```python
from build123d import *

# Parameters (mm, degrees)
EXTRUDE_1_DEPTH     = 10
SKETCH_4_R          = 5.17
CUT_EXTRUDE_1_DEPTH = 10
CHAMFER_1_SIZE      = 0.83


with BuildPart() as part:
    # Эскиз1 → Бобышка-Вытянуть1 (new body)
    with BuildSketch(Plane(origin=(0, 0, 0), x_dir=(1, 0, 0), z_dir=(0, 1, 0))):
        Polygon((-5.484827557, 9.5), (-10.969655115, 0), (-5.484827557, -9.5), (5.484827557, -9.5), (10.969655115, 0), (5.484827557, 9.5), align=None)
    extrude(amount=EXTRUDE_1_DEPTH)

    # Эскиз2 → Вырез-Повернуть1 (revolve, cut)
    with BuildSketch(Plane(origin=(0, 0, 0), x_dir=(0, 0, -1), z_dir=(1, 0, 0))):
        Polygon((-9.5, 10), (-10.97, 10), (-10.97, 9.151295104), align=None)
        Polygon((-9.5, 0), (-10.97, 0), (-10.97, 0.848704896), align=None)
    revolve(axis=Axis((0, -1000, 0), (0, 1, 0)), mode=Mode.SUBTRACT)

    # Эскиз4 → Вырез-Вытянуть1 (cut)
    with BuildSketch(Plane.XZ):
        with Locations(Location((0, 0, 0), (0, 0, 270))):
            Circle(SKETCH_4_R)
    extrude(amount=-CUT_EXTRUDE_1_DEPTH, mode=Mode.SUBTRACT)

    # Фаска1
    chamfer_1_edges = [part.edges().sort_by_distance(p)[0] for p in [
        (0, 10, 5.17),
        (0, 0, 5.17),
    ]]
    chamfer(chamfer_1_edges, length=CHAMFER_1_SIZE)


solid = part.part
```
For this review, take the finished solid that the model builds, in its own axes (mm). Round coordinates to 2 decimals unless told otherwise and drop trailing zeros. Write each loop counter-clockwise with the first axis right and the second up, starting at its lowest first coordinate (ties: lowest second). Pieces come first, ordered by that corner, then holes. Notation, with made-up numbers: (-19, 31.25) -> (-14, 31.25) arc R15 ccw to (-14, 56.25) -> close; hole circle Ø3 at (-1, 4.5). An arc over 180 degrees is marked (long way). One line per question, with ' | ' between items. Start each with the question number.
1) For pin 1 Ø1 at (x, y) = (-8, 1) entering from +Z; pin 2 Ø8 at (x, z) = (-2.5, -1.5) entering from +Y; pin 3 Ø1 at (x, z) = (-3.5, -4) entering from +Y, all flat-tipped, find the tip position at first contact; note any pin that passes through.
2) Add section A-A (y = 1.75). Write out the cut boundary in (x, z), and give its area (3 significant figures).
3) Wall thickness on line 1 along Z through (x, y) = (4, 2); line 2 along X through (y, z) = (7.5, -1); line 3 along X through (y, z) = (3.25, 2.25): over which ranges is each line inside the solid? List them lowest first.
4) Mouldability with a two-part tool opening along Z and no side actions: class faces 1 (the flat face through (-8.2, 4.9, -4.8)), 2 (the flat face through (-8.266, 4.93, 4.684)), 3 (the cylindrical face through (4.36, 4.94, -2.78)) as +Z half, -Z half, draft (parallel to the pull), parting line (faces both ways), or undercut.
Reported:
1) pin 1: stops at z = 6.01 | pin 2: stops at y = 10 | pin 3: stops at y = 9.82
2) outline: (-10.97, 0) -> (-5.48, -9.5) -> (5.48, -9.5) -> (10.97, 0) -> (5.48, 9.5) -> (-5.48, 9.5) -> close; hole circle Ø10.34 at (0, 0) | area: 229 mm²
3) line 1: z = -9.5 to -3.28, 3.28 to 9.5 | line 2: x = -10.39 to -5.07, 5.07 to 10.39 | line 3: x = -9.67 to -4.65, 4.65 to 9.67
4) face 1: -Z half | face 2: +Z half | face 3: undercut
